For this review, use the dimensioned drawing (mm, ordinates from the lowest corner) and the shaded views. A direction names the side the tool comes from. Coordinates: 2 decimals unless noted, no trailing zeros. Loops run counter-clockwise (first coordinate to the right, second up) from the corner with the lowest first, then second, coordinate; pieces in that order, holes last. Notation, with made-up numbers: M 1,-1.5 L 34,-1.5 A18 cw 34,16.5 Z; hole C 81.5,9.25 d10. An arc over 180 degrees is marked long. Write item = value, one per line. Start each with the question number.
Q1. Wall thickness on probe 1 along Z at (x, y) = (7.62, 2.5) (1 decimal); probe 2 along Z at (x, y) = (16.75, 12.5) (1 decimal): over which ranges is each line inside the solid? List them lowest first.
Q2. For the marked faces 4 and 5, list the 3-axis set-ups (+Z, -Z, +X, -X, +Y, -Y) from which the entire face can be reached by the end or side of a thin tool; tool diameter is ignored.
Q3. We need section A-A on x = 7.62. Count the separate pieces of the cut face and the enclosed holes in it.
Q4. Clearance check with flat-ended pins moving along their axes: pin 1 Ø1.5 at (x, z) = (10, 17) entering from +Y (3 decimals); pin 2 Ø4.5 at (x, y) = (7.62, 10.16) entering from +Z (3 decimals). State where each tip first meets the part, or that it passes through.
Q5. We need section D-D on z = 14. Give the boundary of the cut face in (x, y) (1 decimal).
Q6. We need section B-B on y = 20.32. Give the boundary of the cut face in (x, z) (1 decimal).
Q7. Mouldability with a two-part tool opening along X and no side actions: class the marked faces 1, 2 and 3 as released by +X, released by -X, zero draft, split by the parting line, or undercut.
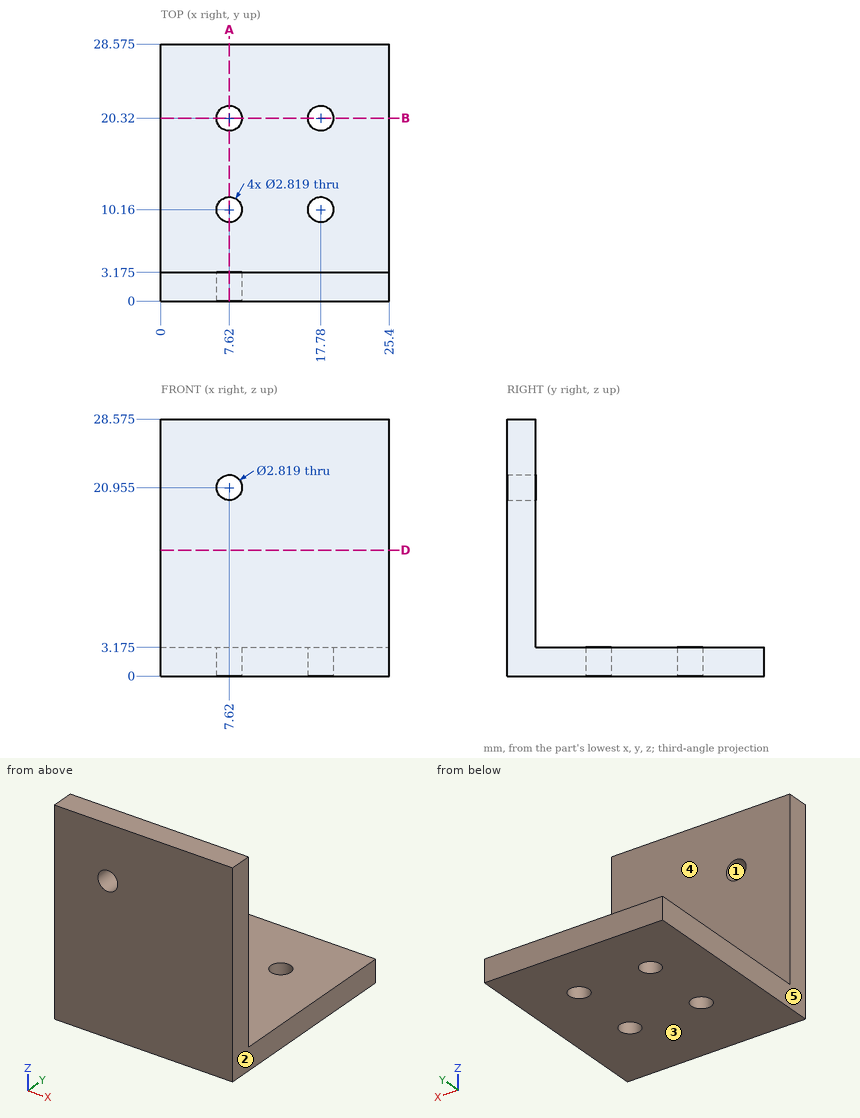
Returned:
q1.probe_1 = 0 to 19.5, 22.4 to 28.6
q1.probe_2 = 0 to 3.2
q2.face_4 = +Z, +X, -X, +Y
q2.face_5 = +Z, -Z, -X, +Y, -Y
q3.separate_pieces = 4
q3.enclosed_holes = 0
q4.pin_1 = 3.175
q4.pin_2 = 3.175
q5.outline = M 0,0 L 25.4,0 L 25.4,3.2 L 0,3.2 Z
q6.outline = M 0,0 L 6.2,0 L 6.2,3.2 L 0,3.2 Z; M 9,0 L 16.4,0 L 16.4,3.2 L 9,3.2 Z; M 19.2,0 L 25.4,0 L 25.4,3.2 L 19.2,3.2 Z
q7.face_1 = undercut
q7.face_2 = released by +X
q7.face_3 = zero draft
